Build history of the part. All positions in model axes, mm. Face numbers are marked on the shaded views. A direction names the side the tool comes from. Give positions to 0.01 mm unless a question says otherwise; leave off trailing zeros. Order: outer loops, then holes, each group sorted by start corner. A loop starts at its lowest first (then second) coordinate and runs counter-clockwise, first axis right, second up. Notation, with made-up numbers: (-39, -13) - (13, -13) arc R13 cw to (13, 1) - close; hole circle Ø5 at (-10.75, 1). An arc over 180 degrees is marked (long way). Use a Markdown table: item, result. Add a question column.
(1) Wall check: line 1 (Y direction, x = 3.5, z = 0.25); line 2 (X direction, y = -3.25, z = -3.25). Give the ranges that are in metal, low to high.
(2) Flat gauge pins, fed straight in: pin 1 (5 mm diameter, centred on x = 80.5, z = 1, fed in from -Y); pin 2 (1.5 mm diameter, centred on y = 0.5, z = 4.5, fed in from +X); pin 3 (8 mm diameter, centred on x = 16.5, y = -2, fed in from -Z). Where does each tip first touch, or does it go through?
(3) Which spindle directions (+Z, -Z, +X, -X, +Y, -Y) get a long thin tool onto all of the face, cutting with end or side? Do the marked faces 1 and 2. Say none if no direction does.
(4) Slice it at A-A (x = 14). Write the cut outline in (y, z), then the cut area to 3 significant figures.
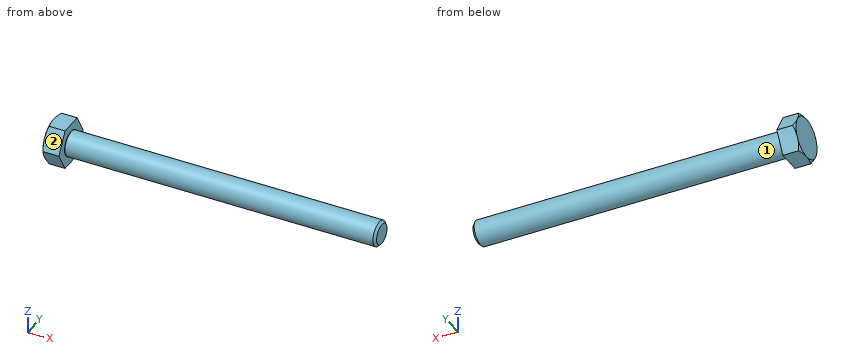
Autodesk Inventor part; units mm, degrees
ref_plane "Work Plane1" through (1.525, 0, 0) normal (0, 0, 1) x (1, 0, 0)
ref_plane "YZ Plane" through (0, 0, 0) normal (1, 0, 0) x (0, 1, 0)
ref_plane "XZ Plane" through (0, 0, 0) normal (0, 1, 0) x (-1, 0, 0)
sketch "Sketch1" plane through (0, 0, 0) normal (0, 0, 1) x (1, 0, 0)
  line L0 (0, 4) -> (100, 4)
  line L1 (100, 4) -> (100, 0)
  line L2 (100, 0) -> (0, 0)
  line L3 (-16, 0) -> (96, 0)
  line L4 (0, -0.8) -> (0, 4.8)
  line L5 (0, 4) -> (0, 0)
  dimension "d2" = 8
  dimension "d59" = 100
revolve "Body" add sketch "Sketch1" angle 360 about axis through (100, 0, 0) along (-1, 0, 0)
sketch "Sketch2" plane through (0, 0, 0) normal (-1, 0, 0) x (0, 0, 1)
  line L0 (0, 7.5056) -> (6.5, 3.7528)
  line L1 (6.5, 3.7528) -> (6.5, -3.7528)
  line L2 (6.5, -3.7528) -> (0, -7.5056)
  line L3 (0, -7.5056) -> (-6.5, -3.7528)
  line L4 (-6.5, -3.7528) -> (-6.5, 3.7528)
  line L5 (-6.5, 3.7528) -> (0, 7.5056)
  line L6 (-9.1, 0) -> (9.1, 0)
  line L7 (0, 10.5078) -> (0, -10.5078)
  point P0 (0, 0)
  point P1 (0, 0)
  dimension "d11" = 13
extrude "Head" add sketch "Sketch2" along normal blind 5.68
sketch "Sketch4" plane through (0, 0, 0) normal (0, 0, 1) x (1, 0, 0)
  line L0 (-4.9294, 7.8) -> (-5.68, 6.5)
  line L1 (-1.1, 0) -> (-0.234, 0)
  line L2 (-6.7692, 0) -> (0.8552, 0)
  line L3 (-5.68, 7.8) -> (-4.9294, 7.8)
  line L4 (-5.68, 6.5) -> (-5.68, 7.8)
  line L5 (0, 9.36) -> (0, -1.56)
  dimension "d65" = 13
  dimension "d67" = 30
  dimension "d68" = 15.6
  dimension "d69" = 5.68
revolve "Chamfer1" cut sketch "Sketch4" angle 360 about axis through (-1.1, 0, 0) along (1, 0, 0)
thread "Thread"
chamfer "Chamfer2" distance 0.7668 distance2 0.7669 1 edges at (100, -4, 0) measured on face at (100, -1.054, 1.6624)
fillet "Fillet" radius 0.1 1 edges at (0, -4, 0)
ref_plane "Work Plane1" through (1.525, 0, 0) normal (0, 0, 1) x (1, 0, 0)
equation "\"d2\" = GD"
equation "\"d59\" = NLG"
equation "\"d11\" = SW"
equation "\"d3\" = KOH"
equation "\"d15\" = GEL"
equation "\"d6\" = -0.5 * SPD + 0.5 * GD"
equation "\"d71\" = RR"
equation "\"d65\" = SW"
equation "\"d67\" = ANG1"
equation "\"d68\" = 1.2 * SW"
equation "\"d69\" = KOH"
equation "\"NLG\" = 100"
equation "\"GD\" = NND"
equation "\"BDM\" = NND"
equation "\"KOH\" = 5.68"
equation "\"GEL\" = 22"
equation "\"SW\" = 13"
equation "\"SW0\" = SW"
equation "\"SPD\" = NND - 1.2269 * PTC"
equation "\"SD2\" = NND"
equation "\"SD\" = 0"
equation "\"ANG1\" = 30deg"
equation "\"GAL\" = 0.61345 * PTC"
equation "\"GUL\" = 0.61345 * PTC"
equation "\"RR\" = 0.1"
equation "\"RR1\" = 0.4"
equation "\"GD1\" = THREADDIA - 1.2269 * PTC"
equation "\"THREADDIA\" = 8"
equation "\"TOA\" = 30deg"
equation "\"PTC\" = 1.25"
equation "\"KOH1\" = 3.7"
equation "\"NND\" = 8"
equation "\"E0\" = 1.155 * SW"
properties material "Steel, Mild"
Solution:
| question | item | result |
|---|---|---|
| 1 | line 1 | -3.99 to 3.99 |
| 1 | line 2 | -5.68 to 0 |
| 2 | pin 1 | y = -4 |
| 2 | pin 2 | x = 99.46 |
| 2 | pin 3 | z = -4 |
| 3 | face 1 | +X |
| 3 | face 2 | +Z, +X, -X, -Y |
| 4 | outline | circle Ø8 at (0, 0) |
| 4 | area | 50.3 mm2 |
